The listing builds one solid part. Answer for the finished solid, in the listing's coordinates (mm). Round coordinates to 2 decimals unless told otherwise and drop trailing zeros. Write each loop counter-clockwise with the first axis right and the second up, starting at its lowest first coordinate (ties: lowest second). Pieces come first, ordered by that corner, then holes. Notation, with made-up numbers: (13.25, 13.25) - (53.25, 13.25) arc R28 ccw to (53.25, 51.25) - close; hole circle Ø5 at (-29.5, 89.5). An arc over 180 degrees is marked (long way). Answer in a Markdown table with one row per item.
from build123d import *

# Parameters (mm, degrees)
F1_DEPTH = 2
F2_R     = 9.5
F3_DEPTH = 25
F6_D     = 3.3


with BuildPart() as f1:
    # F0 (on Front) → F1 (new body)
    with BuildSketch(Plane.XZ):
        Polygon((23, -19), (23, 23), (-23, 23), (-23, -23), (23, -23), align=None)
        Polygon((-23, 23), (23, 23), (0, 27.5), align=None)
        Polygon((23, -23), (-23, -23), (0, -27.5), align=None)
    extrude(amount=F1_DEPTH)

    # F2 (on face) → F3 (cut)
    with BuildSketch(Plane(origin=(0, 0, 0), x_dir=(-1, 0, 0), z_dir=(0, 1, 0))):
        Circle(F2_R)
    extrude(amount=-F3_DEPTH, mode=Mode.SUBTRACT)

    # F6 (through all)
    with Locations(Plane.XZ.offset(2)):
        with Locations((0, -24), (0, 24)):
            Hole(F6_D / 2)


solid = f1.part
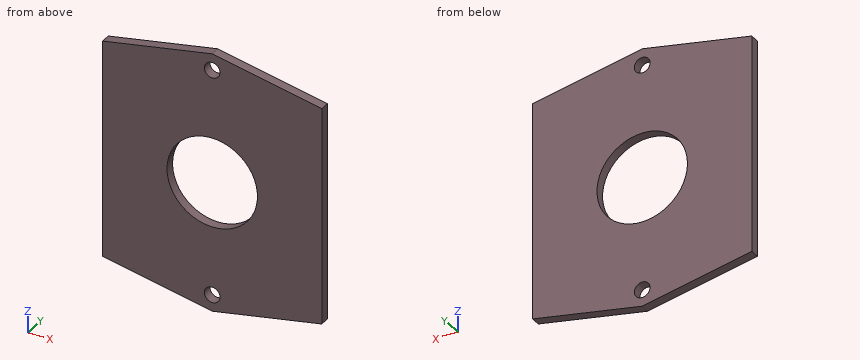
(1) Section B-B (z = 0) is taken. Give the vertices of the cut face in (x, y).
Checked values:
| item | result |
|---|---|
| outline | (-23, -2) - (-9.5, -2) - (-9.5, 0) - (-23, 0) - close; (9.5, -2) - (23, -2) - (23, 0) - (9.5, 0) - close |
(2) Section D-D (z = -24) is taken. Give the vertices of the cut face in (x, y), and give its area (3 significant figures).
Checked values:
| item | result |
|---|---|
| outline | (-17.89, -2) - (-1.65, -2) - (-1.65, 0) - (-17.89, 0) - close; (1.65, -2) - (17.89, -2) - (17.89, 0) - (1.65, 0) - close |
| area | 65.0 mm2 |
(3) Find the intervals of material crossed by line 1 (Z direction, x = 0, y = -0.95); line 2 (X direction, y = -0.2, z = -7); line 3 (Z direction, x = -4, y = -1.45), in increasing order.
Checked values:
| item | result |
|---|---|
| line 1 | z = -27.5 to -25.65, -22.35 to -9.5, 9.5 to 22.35, 25.65 to 27.5 |
| line 2 | x = -23 to -6.42, 6.42 to 23 |
| line 3 | z = -26.72 to -8.62, 8.62 to 26.72 |
(4) Section C-C (x = 11.5) is taken. Give the vertices of the cut face in (y, z).
Checked values:
| item | result |
|---|---|
| outline | (-2, -25.25) - (0, -25.25) - (0, 25.25) - (-2, 25.25) - close |
(5) Section A-A (y = -0.4) is taken. Give the vertices of the cut face in (x, z), and give its area (3 significant figures).
Checked values:
| item | result |
|---|---|
| outline | (-23, -23) - (0, -27.5) - (23, -23) - (23, 23) - (0, 27.5) - (-23, 23) - close; hole circle Ø19 at (0, 0); hole circle Ø3.3 at (0, -24); hole circle Ø3.3 at (0, 24) |
| area | 2,020 mm2 |
(6) A flat-ended cylindrical pin translates along its axis: pin 1 (15 mm diameter, centred on x = 0, z = 0, fed in from +Y). Find the tip coordinate at first contact, or state that the pin passes through.
Checked values:
| item | result |
|---|---|
| pin 1 | passes through |
